Can you work these out from the model? Positions are in its coordinate system, mm. Face numbers are marked on the shaded views. A direction names the side the tool comes from. Give positions to 0.01 mm unless a question says otherwise; leave off trailing zeros. Write each loop counter-clockwise with the first axis right and the second up, starting at its lowest first coordinate (ties: lowest second). Pieces come first, ordered by that corner, then holes. Notation, with made-up numbers: M 74,-28.75 L 89,-28.75 A21 cw 89,-20.75 Z; hole C 23,50.5 d10. An arc over 180 degrees is marked long. Write each question's results on one line, items separated by ' | '.
from build123d import *

# Parameters (mm, degrees)
F1_DEPTH        = 20
F2_R            = 10
F3_R            = 10
F5_R            = 5
F6_R            = 5
F7_R            = 5
F8_R            = 5
F9_R            = 5
F10_R           = 5
F11_R           = 1
F12_R           = 1
F13_R           = 1
F15_D           = 4
F15_CSINK_D     = 7
F15_CSINK_ANGLE = 45
F17_D           = 4
F17_CSINK_D     = 7
F17_CSINK_ANGLE = 45


# Not quite as in the source:
# - two fillets or chamfers of one size are made in one step


with BuildPart() as f1:
    # F0 (on Front) → F1 (new body)
    with BuildSketch(Plane.XZ):
        Polygon((-11.9194036352, -14.2478547741), (13.0805963648, -14.2478547741), (23.7375380173, -3.1786129853), (20.1516641766, 0.305853803), (10.8681305885, -9.2478547741), (-6.9194036352, -9.2478547741), (-6.9194036352, 42.86539388), (59.8626286675, 81.422018207), (57.3626286675, 85.7521452259), (-11.9194036352, 45.7521452259), align=None)
    extrude(amount=F1_DEPTH)

    # F2
    f2_edges = [f1.edges().sort_by_distance(p)[0] for p in [
        (-11.919404, -10, -14.247855),
    ]]
    fillet(f2_edges, radius=F2_R)

    # F3
    f3_edges = [f1.edges().sort_by_distance(p)[0] for p in [
        (-11.919404, -10, 45.752145),
        (13.080596, -10, -14.247855),
    ]]
    fillet(f3_edges, radius=F3_R)

    # F5
    f5_edges = [f1.edges().sort_by_distance(p)[0] for p in [
        (-6.919404, -10, -9.247855),
    ]]
    fillet(f5_edges, radius=F5_R)

    # F6
    f6_edges = [f1.edges().sort_by_distance(p)[0] for p in [
        (-6.919404, -10, 42.865394),
    ]]
    fillet(f6_edges, radius=F6_R)

    # F7
    f7_edges = [f1.edges().sort_by_distance(p)[0] for p in [
        (21.944601, -20, -1.43638),
    ]]
    fillet(f7_edges, radius=F7_R)

    # F8
    f8_edges = [f1.edges().sort_by_distance(p)[0] for p in [
        (21.944601, 0, -1.43638),
    ]]
    fillet(f8_edges, radius=F8_R)

    # F9
    f9_edges = [f1.edges().sort_by_distance(p)[0] for p in [
        (58.612629, -20, 83.587082),
    ]]
    fillet(f9_edges, radius=F9_R)

    # F10
    f10_edges = [f1.edges().sort_by_distance(p)[0] for p in [
        (58.612629, 0, 83.587082),
    ]]
    fillet(f10_edges, radius=F10_R)

    # F11
    f11_edges = [f1.edges().sort_by_distance(p)[0] for p in [
        (25.556549, -20, 61.615394),
    ]]
    fillet(f11_edges, radius=F11_R)

    # F12
    f12_edges = [f1.edges().sort_by_distance(p)[0] for p in [
        (18.150256, -20, -8.982058),
    ]]
    fillet(f12_edges, radius=F12_R)

    # F13
    f13_edges = [f1.edges().sort_by_distance(p)[0] for p in [
        (13.767664, -20, -6.263937),
        (13.767664, 0, -6.263937),
        (19.131087, -1.464466, -0.744424),
        (19.131087, -18.535534, -0.744424),
        (20.151664, -10, 0.305854),
    ]]
    fillet(f13_edges, radius=F13_R)

    # F15 (through all)
    with Locations(Plane.YZ.offset(-6.9194036352)):
        with Locations((-13, 29.978642534)):
            CounterSinkHole(F15_D / 2, F15_CSINK_D / 2, counter_sink_angle=F15_CSINK_ANGLE)

    # F17 (through all)
    with Locations(Plane.YZ.offset(-6.9194036352)):
        with Locations((-7, 15.7521452259)):
            CounterSinkHole(F17_D / 2, F17_CSINK_D / 2, counter_sink_angle=F17_CSINK_ANGLE)


solid = f1.part
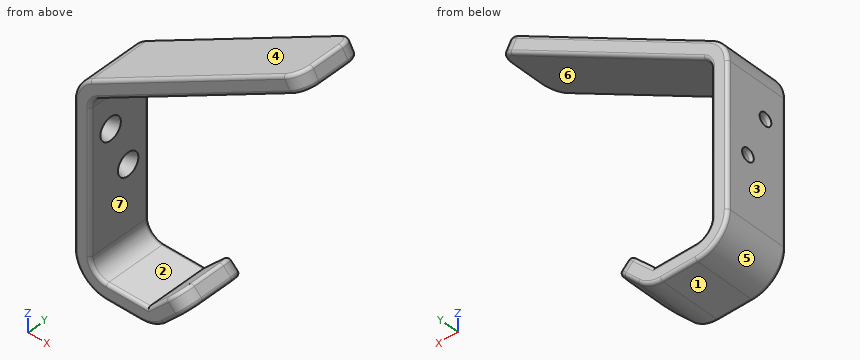
Item 1: I want a section at A-A, the plane y = -13. Please give me the cut outline in (x, z).
Geometry says:
outline: M -11.92,-4.25 A10 ccw -1.92,-14.25 L 8.83,-14.25 A10 ccw 16.03,-11.18 L 23.05,-3.9 A1 ccw 23.02,-2.48 L 20.87,-0.39 A1 ccw 19.45,-0.41 L 10.87,-9.25 L -1.92,-9.25 A5 cw -6.92,-4.25 L -6.92,26.48 L -10.54,27.98 L -11.92,27.98 Z; M -11.92,31.98 L -10.54,31.98 L -6.92,33.48 L -6.92,39.98 A5 cw -4.42,44.31 L 59,80.92 A1 ccw 59.36,82.29 L 57.86,84.89 A1 ccw 56.5,85.25 L -6.92,48.64 A10 ccw -11.92,39.98 Z
Item 2: I'm going to push flat-ended pins straight in: pin 1 (1.5 mm diameter, centred on x = 8.5, y = -7, fed in from +Z); pin 2 (2 mm diameter, centred on x = 10.5, y = -12.5, fed in from -Z); pin 3 (1 mm diameter, centred on y = -7.5, z = 9, fed in from +X); pin 4 (5 mm diameter, centred on x = 26, z = 0, fed in from +Y). Where does each tip first touch, or does it pass through?
Geometry says:
pin 1: stops at z = 57.97 | pin 2: stops at z = -14.23 | pin 3: stops at x = -6.92 | pin 4: passes through
Item 3: I want a section at B-B, the plane z = 1.5. Please give me the cut outline in (x, y).
Geometry says:
outline: M -11.92,-19 A1 ccw -10.92,-20 L -7.92,-20 A1 ccw -6.92,-19 L -6.92,-1 A1 ccw -7.92,0 L -10.92,0 A1 ccw -11.92,-1 Z
Item 4: Thinking about a two-plate mould opening in Z: for the marked faces 1, 2, 3 and 4, which applies, +Z half, -Z half, draft (parallel to the pull), parting line (faces both ways), or undercut?
Geometry says:
face 1: -Z half | face 2: undercut | face 3: draft | face 4: +Z half
Item 5: If I drill on line 1 (X direction, y = -13.25, z = -5); line 2 (X direction, y = -18.75, z = -2); line 3 (Z direction, x = 20.5, y = -12.5), over which ranges is the centre line in solid material (lowest first)? Write a range as from..to.
Geometry says:
line 1: x = -11.89..-6.86, 15..21.98 | line 2: x = -11.92..-6.92, 17.93..20.1 | line 3: z = -6.54..-0.16, 58.7..64.47
Item 6: For the marked faces 5, 6 and 7, which set-ups out of +Z, -Z, +X, -X, +Y, -Y let a thin tool reach every point of the face, with its end or its side?
Geometry says:
face 5: -Z, -X, +Y, -Y | face 6: +X, +Y, -Y | face 7: +Y, -Y
